Model file for the job. Use its own axes, mm. Round coordinates to 2 decimals unless told otherwise and drop trailing zeros. Loops run counter-clockwise (first coordinate to the right, second up) from the corner with the lowest first, then second, coordinate; pieces in that order, holes last. Notation, with made-up numbers: M -32.75,-17 L 1.25,-17 A17 ccw 1.25,-8 Z; hole C 22.25,87 d5. An arc over 180 degrees is marked long. Use a Markdown table: item, result. Add a question column.
Item 1: Wall check: L1, parallel to X at y = 5.5, z = 0; L2, parallel to Z at x = 23.5, y = 0.75; L3, parallel to Z at x = 6, y = 4. Give the ranges that are in metal, low to high. Write a range as from..to.
Item 2: Saw through at B-B on x = 67. Write the cut outline in (y, z), then the cut area to 4 significant figures.
Item 3: Saw through at C-C on x = 38.5. Write the cut outline in (y, z).
Item 4: Saw through at A-A on x = 50. Write the cut outline in (y, z), then the cut area to 3 significant figures.
Item 5: Pin check, flat tips, straight feed: P1, Ø4, axis at x = 85, z = 0, coming from the -Y side; P2, Ø2, axis at x = 94.5, z = 13.5, coming from the +Y side. Stop position of each tip, or through.
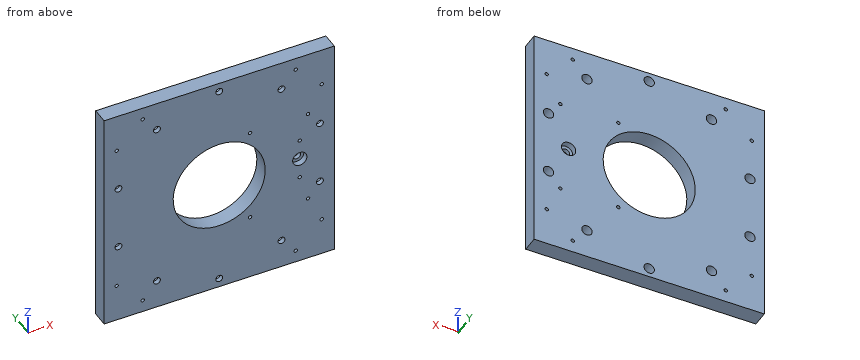
```python
from build123d import *

# Parameters (mm, degrees)
SKETCH_1_W               = 100
SKETCH_1_H               = 100
SKETCH_1_R               = 1.75
SKETCH_1_R_2             = 20
EXTRUDE_1_DEPTH          = 7
CUT_EXTRUDE_START        = 7
SKETCH_1_15_R            = 3.1
CUT_EXTRUDE_2_DEPTH      = 2.6
CUT_EXTRUDE_START_2      = 2.6
SKETCH_1_16_R            = 3.1
CUT_EXTRUDE_3_DEPTH      = 2.6
SKETCH_1_17_R            = 1.5
CUT_EXTRUDE_4_DEPTH      = 113.022319205
SKETCH_1_18_R            = 2.25
CUT_EXTRUDE_5_DEPTH      = 5
PATTERN_CIRCULAR_1_COUNT = 10
SKETCH_2_R               = 0.75
CUT_EXTRUDE_6_DEPTH      = 4
SKETCH_3_R               = 0.75
CUT_EXTRUDE_7_DEPTH      = 113.022319205
PATTERN_CIRCULAR_2_COUNT = 4
SKETCH_3_3_R             = 0.75
CUT_EXTRUDE_8_DEPTH      = 113.022319205


with BuildPart() as part:
    # 草图1 → 凸台-拉伸1 (new body)
    with BuildSketch(Plane(origin=(0, 0, 0), x_dir=(1, 0, 0), z_dir=(0, 1, 0))):
        with Locations((50, 0)):
            Rectangle(SKETCH_1_W, SKETCH_1_H)
        with Locations(Location((85, 0, 0), (0, 0, 270))):
            Circle(SKETCH_1_R, mode=Mode.SUBTRACT)
        with Locations(Location((50, 0, 0), (0, 0, 270))):
            Circle(SKETCH_1_R_2, mode=Mode.SUBTRACT)
    extrude(amount=EXTRUDE_1_DEPTH)

    # 草图1<15> → 切除-拉伸2 (cut)
    with BuildSketch(Plane(origin=(0, 0, 0), x_dir=(1, 0, 0), z_dir=(0, 1, 0)).offset(CUT_EXTRUDE_START)):
        with Locations(Location((85, 0, 0), (0, 0, 270))):
            Circle(SKETCH_1_15_R)
    extrude(amount=-CUT_EXTRUDE_2_DEPTH, mode=Mode.SUBTRACT)

    # 草图1<16> → 切除-拉伸3 (cut)
    with BuildSketch(Plane(origin=(0, 0, 0), x_dir=(1, 0, 0), z_dir=(0, 1, 0)).offset(CUT_EXTRUDE_START_2)):
        with Locations(Location((85, 0, 0), (0, 0, 270))):
            Circle(SKETCH_1_16_R)
    extrude(amount=-CUT_EXTRUDE_3_DEPTH, mode=Mode.SUBTRACT)

    # 草图1<17> → 切除-拉伸4 (cut, through all)
    with BuildSketch(Plane(origin=(0, 0, 0), x_dir=(1, 0, 0), z_dir=(0, 1, 0))):
        with Locations(Location((50, 46, 0), (0, 0, 270))):
            Circle(SKETCH_1_17_R)
    cut_extrude_4 = extrude(amount=CUT_EXTRUDE_4_DEPTH, mode=Mode.SUBTRACT)

    # 草图1<18> → 切除-拉伸5 (cut)
    with BuildSketch(Plane(origin=(0, 0, 0), x_dir=(1, 0, 0), z_dir=(0, 1, 0)).offset(CUT_EXTRUDE_START)):
        with Locations(Location((50, 46, 0), (0, 0, 270))):
            Circle(SKETCH_1_18_R)
    cut_extrude_5 = extrude(amount=-CUT_EXTRUDE_5_DEPTH, mode=Mode.SUBTRACT)

    # 阵列(圆周)1: 切除-拉伸4, 切除-拉伸5 ×10 about axis
    pattern_circular_1_axis = Axis((50, 0, 0), (0, 1, 0))
    add([cut_extrude_4.rotate(pattern_circular_1_axis, i * 360 / PATTERN_CIRCULAR_1_COUNT) for i in range(1, PATTERN_CIRCULAR_1_COUNT)], mode=Mode.SUBTRACT)
    add([cut_extrude_5.rotate(pattern_circular_1_axis, i * 360 / PATTERN_CIRCULAR_1_COUNT) for i in range(1, PATTERN_CIRCULAR_1_COUNT)], mode=Mode.SUBTRACT)

    # 草图2 → 切除-拉伸6 (cut)
    with BuildSketch(Plane.XZ):
        with Locations(Location((85, 9, 0), (0, 0, 270))):
            Circle(SKETCH_2_R)
        with Locations(Location((85, -9, 0), (0, 0, 270))):
            Circle(SKETCH_2_R)
    extrude(amount=-CUT_EXTRUDE_6_DEPTH, mode=Mode.SUBTRACT)

    # 草图3 → 切除-拉伸7 (cut, through all)
    with BuildSketch(Plane(origin=(0, 7, 0), x_dir=(1, 0, 0), z_dir=(0, 1, 0))):
        with Locations(Location((5.452272785, 33.234018716, 0), (0, 0, 270))):
            Circle(SKETCH_3_R)
        with Locations(Location((16.765981284, 44.547727215, 0), (0, 0, 270))):
            Circle(SKETCH_3_R)
    cut_extrude_7 = extrude(amount=-CUT_EXTRUDE_7_DEPTH, mode=Mode.SUBTRACT)

    # 阵列(圆周)2: 切除-拉伸7 ×4 about axis
    pattern_circular_2_axis = Axis((50, 0, 0), (0, 1, 0))
    for i in range(1, PATTERN_CIRCULAR_2_COUNT):
        add(cut_extrude_7.rotate(pattern_circular_2_axis, i * 360 / PATTERN_CIRCULAR_2_COUNT), mode=Mode.SUBTRACT)

    # 草图3<3> → 切除-拉伸8 (cut, through all)
    with BuildSketch(Plane(origin=(0, 7, 0), x_dir=(1, 0, 0), z_dir=(0, 1, 0))):
        with Locations(Location((63.404969626, 20.785281374, 0), (0, 0, 270))):
            Circle(SKETCH_3_3_R)
        with Locations(Location((88.584828776, 20.785281374, 0), (0, 0, 270))):
            Circle(SKETCH_3_3_R)
        with Locations(Location((63.404969626, -20.714718626, 0), (0, 0, 270))):
            Circle(SKETCH_3_3_R)
        with Locations(Location((88.584828776, -20.714718626, 0), (0, 0, 270))):
            Circle(SKETCH_3_3_R)
    extrude(amount=-CUT_EXTRUDE_8_DEPTH, mode=Mode.SUBTRACT)


solid = part.part
```
Entries:
| question | item | result |
|---|---|---|
| 1 | L1 | 0..30, 70..81.9, 88.1..100 |
| 1 | L2 | -50..-38.61, -35.81..35.81, 38.61..50 |
| 1 | L3 | -50..-33.75, -32.72..-16.45, -11.98..11.98, 16.45..32.72, 33.75..50 |
| 2 | outline | M 0,-50 L 7,-50 L 7,-10.54 L 0,-10.54 Z; M 0,10.54 L 7,10.54 L 7,50 L 0,50 Z |
| 2 | area | 552.5 mm2 |
| 3 | outline | M 0,-50 L 7,-50 L 7,-16.36 L 0,-16.36 Z; M 0,16.36 L 7,16.36 L 7,50 L 0,50 Z |
| 4 | outline | M 0,-50 L 7,-50 L 7,-48.25 L 2,-48.25 L 2,-47.5 L 0,-47.5 Z; M 0,-44.5 L 2,-44.5 L 2,-43.75 L 7,-43.75 L 7,-20 L 0,-20 Z; M 0,20 L 7,20 L 7,43.75 L 2,43.75 L 2,44.5 L 0,44.5 Z; M 0,47.5 L 2,47.5 L 2,48.25 L 7,48.25 L 7,50 L 0,50 Z |
| 4 | area | 363 mm2 |
| 5 | P1 | y = 2.6 |
| 5 | P2 | y = 2 |
